Could you check a few things on this model? Use its own coordinates, in mm. A direction names the side the tool comes from. Give positions to 0.01 mm unless a question says otherwise; leave off trailing zeros. Order: outer loops, then holes, each group sorted by start corner. A loop starts at its lowest first (then second) coordinate and runs counter-clockwise, first axis right, second up. Notation, with made-up numbers: M -19.5,8 L -13.5,8 A21 cw -13.5,39 Z; hole C 10,18 d10. An arc over 180 degrees is marked long. Return JSON: item names as keys, results as strings. Group by question number.
Autodesk Inventor part; units mm, degrees
ref_plane "YZ Plane" through (0, 0, 0) normal (1, 0, 0) x (0, 1, 0)
ref_plane "XZ Plane" through (0, 0, 0) normal (0, 1, 0) x (-1, 0, 0)
ref_plane "XY Plane" through (0, 0, 0) normal (0, 0, 1) x (1, 0, 0)
sketch "Sketch1" plane through (0, 0, 0) normal (0, 1, 0) x (-1, 0, 0)
  line L0 (-25, 89) -> (25, 89)
  line L1 (25, 89) -> (25, -89)
  line L2 (25, -89) -> (-25, -89)
  line L3 (-25, -89) -> (-25, 89)
  line L4 (-25, 89) -> (25, -89) construction
  line L5 (25, 89) -> (-25, -89) construction
  point P0 (0, 0)
  dimension "d0" = 178
  dimension "d1" = 50
extrude "Extrusion1" add sketch "Sketch1" along normal blind 177
sketch "Sketch2" plane through (0, 177, 0) normal (0, 1, 0) x (1, 0, 0)
  line L0 (27, -91) -> (-27, -91)
  line L1 (-27, -91) -> (-27, 91)
  line L2 (-27, 91) -> (27, 91)
  line L3 (27, 91) -> (27, -91)
  line L4 (27, -91) -> (-27, 91) construction
  line L5 (-27, -91) -> (27, 91) construction
  line L6 (25, 89) -> (-25, 89)
  line L7 (-25, 89) -> (-25, -89)
  point P0 (0, 0)
  dimension "d4" = 2
  dimension "d5" = 2
extrude "Extrusion2" add sketch "Sketch2" along normal blind 2
sketch "Sketch3" plane through (0, 179, 0) normal (0, 1, 0) x (1, 0, 0)
  line L0 (-28.0615, -91.1516) -> (-28.0615, 90.8484) construction
  line L1 (-28.0615, 90.8484) -> (28.3189, 90.8484) construction
  line L2 (28.3189, 90.8484) -> (28.3189, -91.1516) construction
  line L3 (28.3189, -91.1516) -> (-28.0615, -91.1516) construction
equation "\"d0\" = l_stereo"
equation "\"d1\" = w_stereo"
equation "\"d2\" = d_stereo"
equation "\"d5\" = d4"
equation "\"wl_panel\" = 285"
equation "\"t_panel\" = 8"
equation "\"r_button\" = 8"
equation "\"l_stereo\" = 178"
equation "\"w_stereo\" = 50"
equation "\"d_stereo\" = 177"
equation "\"w_label\" = 15"
equation "\"r_labelscrew\" = 2.5"
equation "\"ro_labelscrew\" = 5"
equation "\"l_buttontobutton\" = 25"
equation "\"r_usboutlet\" = 29"
equation "\"l_fastener_button\" = 19"
properties part number "stereo" material "Stainless Steel"
1. I need wall thicknesses on L1, parallel to X at y = 55, z = -17.5; L2, parallel to Z at x = -16.5, y = 43. Which ranges of each line are inside material? Lowest first, please. Write a range as from..to.
2. For pin 1 (6 mm diameter, centred on x = -5, y = 153, fed in from -Z); pin 2 (3 mm diameter, centred on y = 159.5, z = -14, fed in from -X); pin 3 (12 mm diameter, centred on x = 10, y = 134, fed in from +Z), each with a flat end and sliding along its axis, tell me the tip position at first contact or that it passes through.
3. Imagine slicing it at A-A, the plane x = 2.5. Please give me the cut outline in (y, z), plus the area to 3 significant figures.
4. Imagine slicing it at B-B, the plane z = 36. Please give me the cut outline in (x, y).
5. Which directions (+Z, -Z, +X, -X, +Y, -Y) give clear straight access to the entire face, cutting with the end or side of a thin tool? Please do faces 1 (the flat face through (25, 87, -1)), 2 (the flat face through (-25, 87, 1)), 3 (the flat face through (0, 0, 1)), 4 (the flat face through (0, 87, -89)), 5 (the flat face through (0, 87, 89)).
6. Imagine slicing it at C-C, the plane y = 123.5. Please give me the cut outline in (x, z), plus the area to 3 significant figures.
Values:
{
 "1": {"L1": "x = -25..25", "L2": "z = -89..89"},
 "2": {"pin 1": "stops at z = -89", "pin 2": "stops at x = -25", "pin 3": "stops at z = 89"},
 "3": {"outline": "M 0,-89 L 177,-89 L 177,-91 L 179,-91 L 179,91 L 177,91 L 177,89 L 0,89 Z", "area": "31,900 mm²"},
 "4": {"outline": "M -27,177 L -25,177 L -25,0 L 25,0 L 25,177 L 27,177 L 27,179 L -27,179 Z"},
 "5": {"face 1": "+Z, -Z, +X, -Y", "face 2": "+Z, -Z, -X, -Y", "face 3": "+Z, -Z, +X, -X, -Y", "face 4": "-Z, +X, -X, -Y", "face 5": "+Z, +X, -X, -Y"},
 "6": {"outline": "M -25,-89 L 25,-89 L 25,89 L -25,89 Z", "area": "8,900 mm²"}
}
